```python
from build123d import *

# Parameters (mm, degrees)
SKETCH1_W           = 16.002
SKETCH1_H           = 38.1
BOSS_EXTRUDE1_DEPTH = 3.175
SKETCH2_W           = 16.002
SKETCH2_H           = 3.175
BOSS_EXTRUDE2_DEPTH = 38.1
SKETCH3_R           = 3.175
CUT_EXTRUDE1_DEPTH  = 56.143781701
SKETCH4_R           = 3.175
CUT_EXTRUDE2_DEPTH  = 56.235109172
CHAMFER1_SIZE       = 1.190625
FILLET1_R           = 1.190625


with BuildPart() as part:
    # Sketch1 → Boss-Extrude1 (new body)
    with BuildSketch(Plane(origin=(0, 0, 0), x_dir=(1, 0, 0), z_dir=(0, 1, 0))):
        with Locations((8.001, 19.05)):
            Rectangle(SKETCH1_W, SKETCH1_H)
    extrude(amount=BOSS_EXTRUDE1_DEPTH)

    # Sketch2 → Boss-Extrude2 (add)
    with BuildSketch(Plane.XZ):
        with Locations((8.001, -38.1)):
            Rectangle(SKETCH2_W, SKETCH2_H)
    extrude(amount=-BOSS_EXTRUDE2_DEPTH)

    # Sketch3 → Cut-Extrude1 (cut, through all)
    with BuildSketch(Plane.XY.offset(-36.5125)):
        with Locations((9.652, 30.1625)):
            Circle(SKETCH3_R)
        with Locations((6.35, 15.875)):
            Circle(SKETCH3_R)
    extrude(amount=-CUT_EXTRUDE1_DEPTH, mode=Mode.SUBTRACT)

    # Sketch4 → Cut-Extrude2 (cut, through all)
    with BuildSketch(Plane(origin=(0, 3.175, 0), x_dir=(1, 0, 0), z_dir=(0, 1, 0))):
        with Locations(Location((9.652, 22.225, 0), (0, 0, 270))):
            Circle(SKETCH4_R)
        with Locations(Location((6.35, 7.9375, 0), (0, 0, 270))):
            Circle(SKETCH4_R)
    extrude(amount=-CUT_EXTRUDE2_DEPTH, mode=Mode.SUBTRACT)

    # Chamfer1
    chamfer1_edges = [part.edges().sort_by_distance(p)[0] for p in [
        (6.477, 30.1625, -36.5125),
        (3.175, 15.875, -36.5125),
        (9.652, 3.175, -25.4),
        (6.35, 3.175, -11.1125),
    ]]
    chamfer(chamfer1_edges, length=CHAMFER1_SIZE)

    # Fillet1
    fillet1_edges = [part.edges().sort_by_distance(p)[0] for p in [
        (16.002, 3.175, -18.25625),
        (0, 3.175, -18.25625),
        (8.001, 0, -39.6875),
        (8.001, 38.1, -36.5125),
        (0, 20.6375, -36.5125),
        (16.002, 20.6375, -36.5125),
        (8.001, 3.175, -36.5125),
        (8.001, 3.175, 0),
    ]]
    fillet(fillet1_edges, radius=FILLET1_R)


solid = part.part
```
Geometry check sheet. Reference: the model listing, model coordinates, mm. A direction names the side the tool comes from. Give positions to 0.01 mm unless a question says otherwise; leave off trailing zeros. Write each loop counter-clockwise with the first axis right and the second up, starting at its lowest first coordinate (ties: lowest second). Pieces come first, ordered by that corner, then holes.
1) Section check C-C, the plane x = 7. State how many separate pieces and enclosed holes the cut face has, and give its area (3 significant figures).
2) Material ranges on L1, parallel to Y at x = 14.5, z = -31 (3 decimals); L2, parallel to Y at x = 6.35, z = -39.1; L3, parallel to Y at x = 6.35, z = -39, recorded low to high.
3) Access from +Z, -Z, +X, -X, +Y, -Y to the whole of each face (thin tool, end or side, straight path). Record for faces 4 (the cylindrical face through (15.64, 2.84, -17.91)), 5 (the cylindrical face through (0.36, 2.84, -17.91)), 6 (the flat face through (7.9, 20.4, -36.512)).
4) Gauge pin test, flat ends, axial feed: pin 1 (7 mm diameter, centred on x = 10.5, z = -21.5, fed in from +Y) (3 decimals); pin 2 (6 mm diameter, centred on x = 7.5, y = 20, fed in from +Z). Record the tip position at first contact, or that the pin passes through.
5) Release check for a two-part mould opening along X. For faces 1 (the cylindrical face through (3.178, 16.015, -38.681)), 2 (the cylindrical face through (8.11, 2.84, -0.36)), 3 (the cylindrical face through (15.64, 21.47, -36.85)) record: pulls with the +X half, pulls with the -X half, needs draft (parallel to the pull), parting line crosses it, or undercut.
6) Section check B-B, the plane y = 36. Record the boundary of the cut face in (x, z), and give its area (3 significant figures).
7) Section check A-A, the plane z = -16. Record the boundary of the cut face in (x, y) (3 decimals), and give its area (3 significant figures).
Computed:
1. separate pieces: 5
1. enclosed holes: 0
1. area: 167 mm2
2. L1: y = 0 to 3.175
2. L2: y = 0.16 to 12.7, 19.05 to 38.1
2. L3: y = 0.11 to 12.7, 19.05 to 38.1
3. face 4: +Z, +X, +Y
3. face 5: +Z, -X, +Y
3. face 6: +Z, +X, -X, +Y
4. pin 1: stops at y = 3.175
4. pin 2: stops at z = -36.51
5. face 1: undercut
5. face 2: needs draft
5. face 3: pulls with the +X half
6. outline: (0, -39.69) - (16, -39.69) - (16, -37.7) arc R1.19 ccw to (14.81, -36.51) - (1.19, -36.51) arc R1.19 ccw to (0, -37.7) - close
6. area: 50.2 mm2
7. outline: (0, 0) - (16.002, 0) - (16.002, 1.984) arc R1.191 ccw to (14.811, 3.175) - (1.191, 3.175) arc R1.191 ccw to (0, 1.984) - close
7. area: 50.2 mm2
